from build123d import *

# Parameters (mm, degrees)
IZIM4_R                     = 145
IZIM5_W                     = 360
IZIM5_H                     = 360
Y_KSEKLIK_EKSTR_ZYON1_DEPTH = 50
IZIM6_W                     = 360
IZIM6_H                     = 360
Y_KSEKLIK_EKSTR_ZYON2_DEPTH = 50
IZIM7_R                     = 15
KES_EKSTR_ZYON1_DEPTH       = 50
IZIM8_R                     = 30
KES_EKSTR_ZYON2_DEPTH       = 10
IZIM9_R                     = 15
Y_KSEKLIK_EKSTR_ZYON3_DEPTH = 50
IZIM9_2_R                   = 15
KES_EKSTR_ZYON3_DEPTH       = 50
IZIM10_R                    = 30
KES_EKSTR_ZYON4_DEPTH       = 10
KES_S_P_R2_PROFILE_R        = 105
IZIM47_R                    = 105
KES_EKSTR_ZYON5_DEPTH       = 50
IZIM48_R                    = 105
KES_EKSTR_ZYON6_DEPTH       = 50


with BuildPart() as part:
    # S_p_r1: sweep along a path in izim1
    with BuildLine(Plane.XY) as s_p_r1_path:
        Line((0, 0), (-150, 0))
        ThreePointArc((-150, 0), (-333.847763109, 76.152236891), (-410, 260))
        Line((-410, 260), (-410, 410))
    # izim4 → S_p_r1 (sweep)
    with BuildSketch(Plane(origin=(0, 0, 0), x_dir=(0, 0, -1), z_dir=(1, 0, 0))):
        Circle(IZIM4_R)
    sweep(path=s_p_r1_path.line)

    # izim5 → Y_kseklik-Ekstr_zyon1 (add)
    with BuildSketch(Plane(origin=(0, 410, 0), x_dir=(1, 0, 0), z_dir=(0, 1, 0))):
        with Locations((-410, 0)):
            Rectangle(IZIM5_W, IZIM5_H)
    extrude(amount=-Y_KSEKLIK_EKSTR_ZYON1_DEPTH)

    # izim6 → Y_kseklik-Ekstr_zyon2 (add)
    with BuildSketch(Plane(origin=(0, 0, 0), x_dir=(0, 0, -1), z_dir=(1, 0, 0))):
        Rectangle(IZIM6_W, IZIM6_H)
    extrude(amount=-Y_KSEKLIK_EKSTR_ZYON2_DEPTH)

    # izim7 → Kes-Ekstr_zyon1 (cut)
    with BuildSketch(Plane(origin=(0, 410, 0), x_dir=(1, 0, 0), z_dir=(0, 1, 0))):
        with Locations((-540, 130)):
            Circle(IZIM7_R)
        with Locations((-280, 130)):
            Circle(IZIM7_R)
        with Locations((-540, -130)):
            Circle(IZIM7_R)
        with Locations((-280, -130)):
            Circle(IZIM7_R)
    extrude(amount=-KES_EKSTR_ZYON1_DEPTH, mode=Mode.SUBTRACT)

    # izim8 → Kes-Ekstr_zyon2 (cut)
    with BuildSketch(Plane(origin=(0, 410, 0), x_dir=(1, 0, 0), z_dir=(0, 1, 0))):
        with Locations((-540, 130)):
            Circle(IZIM8_R)
        with Locations((-280, 130)):
            Circle(IZIM8_R)
        with Locations((-280, -130)):
            Circle(IZIM8_R)
        with Locations((-540, -130)):
            Circle(IZIM8_R)
    extrude(amount=-KES_EKSTR_ZYON2_DEPTH, mode=Mode.SUBTRACT)

    # izim9 → Y_kseklik-Ekstr_zyon3 (add)
    with BuildSketch(Plane(origin=(0, 0, 0), x_dir=(0, 0, -1), z_dir=(1, 0, 0))):
        with Locations((-130, 130)):
            Circle(IZIM9_R)
        with Locations((130, 130)):
            Circle(IZIM9_R)
        with Locations((130, -130)):
            Circle(IZIM9_R)
        with Locations((-130, -130)):
            Circle(IZIM9_R)
    extrude(amount=-Y_KSEKLIK_EKSTR_ZYON3_DEPTH)

    # izim9_2 → Kes-Ekstr_zyon3 (cut)
    with BuildSketch(Plane(origin=(0, 0, 0), x_dir=(0, 0, -1), z_dir=(1, 0, 0))):
        with Locations((-130, 130)):
            Circle(IZIM9_2_R)
        with Locations((130, 130)):
            Circle(IZIM9_2_R)
        with Locations((130, -130)):
            Circle(IZIM9_2_R)
        with Locations((-130, -130)):
            Circle(IZIM9_2_R)
    extrude(amount=-KES_EKSTR_ZYON3_DEPTH, mode=Mode.SUBTRACT)

    # izim10 → Kes-Ekstr_zyon4 (cut)
    with BuildSketch(Plane(origin=(0, 0, 0), x_dir=(0, 0, -1), z_dir=(1, 0, 0))):
        with Locations((-130, 130)):
            Circle(IZIM10_R)
        with Locations((130, 130)):
            Circle(IZIM10_R)
        with Locations((130, -130)):
            Circle(IZIM10_R)
        with Locations((-130, -130)):
            Circle(IZIM10_R)
    extrude(amount=-KES_EKSTR_ZYON4_DEPTH, mode=Mode.SUBTRACT)

    # Kes-S_p_r2: sweep along a path in izim11
    with BuildLine(Plane.XY) as kes_s_p_r2_path:
        Line((-50, 0), (-150, 0))
        ThreePointArc((-150, 0), (-333.847763109, 76.152236891), (-410, 260))
        Line((-410, 260), (-410, 360))
    # Kes-S_p_r2 profile (on start of the path) → Kes-S_p_r2 (sweep, cut)
    with BuildSketch(Plane(origin=(-50, 0, 0), x_dir=(0, -1, 0), z_dir=(-1, 0, 0))):
        Circle(KES_S_P_R2_PROFILE_R)
    sweep(path=kes_s_p_r2_path.line, mode=Mode.SUBTRACT)

    # izim47 → Kes-Ekstr_zyon5 (cut)
    with BuildSketch(Plane(origin=(0, 0, 0), x_dir=(0, 0, -1), z_dir=(1, 0, 0))):
        Circle(IZIM47_R)
    extrude(amount=-KES_EKSTR_ZYON5_DEPTH, mode=Mode.SUBTRACT)

    # izim48 → Kes-Ekstr_zyon6 (cut)
    with BuildSketch(Plane(origin=(0, 410, 0), x_dir=(1, 0, 0), z_dir=(0, 1, 0))):
        with Locations((-410, 0)):
            Circle(IZIM48_R)
    extrude(amount=-KES_EKSTR_ZYON6_DEPTH, mode=Mode.SUBTRACT)


solid = part.part
Verification items for the finished model (mm, model axes). A direction names the side the tool comes from. Coordinates: 2 decimals unless noted, no trailing zeros. Order: outer loops, then holes, each group sorted by start corner. A loop starts at its lowest first (then second) coordinate and runs counter-clockwise, first axis right, second up. Notation, with made-up numbers: M 14.5,35 L 32.5,35 A27 cw 32.5,54 Z; hole C 7.25,22.25 d5. An arc over 180 degrees is marked long. One line per item, written item: value. Start each with the question number.
Item 1: Depth check by flat-ended pin: P1, Ø1, axis at x = -297.5, y = 125, coming from the -Z side; P2, Ø1, axis at x = -218.5, y = -104.5, coming from the +Z side; P3, Ø6, axis at y = 217.5, z = -61, coming from the +X side; P4, Ø18, axis at x = -540, z = -130, coming from the -Y side. Enter the tip coordinate at first touch or a pass-through.
Item 2: Sectioned sample at C-C on z = 76.5. Record the cut outline in (x, y).
Item 3: Sectioned sample at B-B on x = -278.5. Give the number of separate pieces and of enclosed holes in the cut face, then the cut area to 3 significant figures.
Item 4: Sectioned sample at A-A on z = 0. Record the cut outline in (x, y), then the cut area to 3 significant figures.
Item 5: Mould release check, pull along Y, two halves, no side actions. Record for faces 6 (the flat face through (-10, 144, 124)), 7 (the flat face through (-534, 400, -144)), 8 (the flat face through (0, 83, 83)): pulls with the +Y half, pulls with the -Y half, needs draft (parallel to the pull), parting line crosses it, or undercut.
Item 6: Access from +Z, -Z, +X, -X, +Y, -Y to the whole of each face (thin tool, end or side, straight path). Record for faces 1 (the cylindrical face through (-4.93, 100.713, 136.503)), 2 (the cylindrical face through (-532.265, 310.7, -77.951)), 3 (the flat face through (-413, 385, -180)), 4 (the flat face through (-294, 400, 136)), 5 (the flat face through (-25, 180, 3)).
Item 7: Thickness scan on probe 1 along Y at (x, z) = (-34.5, -130); probe 2 along Y at (x, z) = (-128, 0); probe 3 along Y at (x, z) = (-135.5, 12). Record the ranges inside material, lowest first.
Calculated:
1. P1: z = -132.21
1. P2: z = 94.03
1. P3: x = -269.42
1. P4: through
2. outline: M -590,360 L -533.18,360 L -533.18,260 A383.18 ccw -150,-123.18 L -50,-123.18 L -50,-180 L 0,-180 L 0,-71.92 L -150,-71.92 A331.92 cw -481.92,260 L -481.92,410 L -590,410 Z; M -338.08,260 A188.08 ccw -150,71.92 L 0,71.92 L 0,180 L -50,180 L -50,123.18 L -150,123.18 A136.82 cw -286.82,260 L -286.82,360 L -230,360 L -230,410 L -338.08,410 Z
3. separate pieces: 3
3. enclosed holes: 1
3. area: 70,800 mm^2
4. outline: M -590,360 L -555,360 L -555,260 A405 ccw -150,-145 L -50,-145 L -50,-180 L 0,-180 L 0,-105 L -150,-105 A365 cw -515,260 L -515,410 L -590,410 Z; M -305,260 A155 ccw -150,105 L 0,105 L 0,180 L -50,180 L -50,145 L -150,145 A115 cw -265,260 L -265,360 L -230,360 L -230,410 L -305,410 Z
4. area: 63,700 mm^2
5. face 6: undercut
5. face 7: pulls with the +Y half
5. face 8: needs draft
6. face 1: +X
6. face 2: none
6. face 3: -Z, +X, -X, +Y, -Y
6. face 4: +Y
6. face 5: +Z, -Z, +X, +Y
7. probe 1: -180 to -145, -115 to 115, 145 to 180
7. probe 2: -145 to -105, 105 to 145
7. probe 3: -144.5 to -104.31, 104.31 to 144.5
